Input: part model. Units: mm. Frame: model coordinates. A direction names the side the tool comes from. Round coordinates to 2 decimals unless told otherwise and drop trailing zeros. Loops run counter-clockwise (first coordinate to the right, second up) from the corner with the lowest first, then second, coordinate; pieces in that order, holes last. Notation, with made-up numbers: (29, -13.75) -> (83, -13.75) arc R13 ccw to (83, -9.75) -> close; hole circle Ø5 at (27.5, 13). An arc over 180 degrees is marked (long way). Answer as a JSON object with one key per item and string values. Group by question number.
Item 1: Set-up query: faces 1 (the flat face through (-53.68, -18.54, 1.06)), 2 (the flat face through (58, -6, 4.318)), 3 (the flat face through (-42, -6, 4.318)), 4 (the flat face through (58, -6, 0)). Return all of +Z, -Z, +X, -X, +Y, -Y with unobstructed straight access to the full face (end or side cutting, diameter ignored); none if empty.
Item 2: Material intervals for line 1 (Y direction, x = 51, z = 3); line 2 (Z direction, x = -2, y = -6.5); line 3 (X direction, y = -9, z = -0.5), sorted ascending. Write a range as [from, to].
Item 3: Pin query (flat end, axial travel): pin 1 (2 mm diameter, centred on y = -4.5, z = 4.5, fed in from -X); pin 2 (3.5 mm diameter, centred on x = 30.5, z = 2, fed in from -Y); pin 3 (4 mm diameter, centred on x = 8, y = -6.5, fed in from -Z). Return the tip coordinate at first contact, or that it passes through.
Item 4: Section query D-D on x = 54. Return loops of the section in (y, z), and give its area (3 significant figures).
Item 5: Draft query along X for faces 5 (the flat face through (30, -6, 6.096)), 6 (the flat face through (80.004, -11.053, 2.129)), 7 (the flat face through (4.6, -14.04, 1.06)). Return one class per face: released by +X, released by -X, zero draft, split by the parting line, or undercut.
from build123d import *

# Parameters (mm, degrees)
F2_DEPTH = 4.318
F3_SIZE  = 2.15899
F5_DEPTH = 1.778
F7_DEPTH = 1.778
F8_R     = 1.778
F9_SIZE  = 1.778


# Not quite as in the source:
# - a fillet or chamfer is up to 0.001 mm smaller than in the source, because OpenCascade refuses the exact size


with BuildPart() as f2:
    # F0 (on Top) → F2 (new body)
    with BuildSketch(Plane.XY):
        Polygon((27.5745280087, 3.6292271689), (27.5745280087, 1.2858584523), (27.5745280087, -13.2207097486), (27.5745280087, -15.5640784651), (32.4286483228, -15.5640784651), (32.4286483228, -13.3150536567), (32.4286483228, 1.3802023605), (32.4286483228, 3.6292271689), align=None)
        Polygon((72.2789242864, 1.3802023605), (32.4286483228, 1.3802023605), (32.4286483228, -13.3150536567), (72.2789242864, -13.3150536567), (75.0406160951, -15.9978345037), (85.1087123156, -5.9674256481), (75.0406160951, 4.0629832074), align=None)
        Polygon((-64.9878308177, 19.7724616155), (-86.7510214448, 19.7724616155), (-86.7510214448, -31.7073129117), (-64.9878308177, -31.7073129117), (-64.9878308177, -20.5603092909), (-42.1630144119, -18.7024753541), (-42.1630144119, -31.7073129117), (-15.7552305609, -31.7073129117), (-15.7552305609, -16.8446414173), (27.5745280087, -13.2207097486), (27.5745280087, 1.2858584523), (-15.7552305609, 4.909790121), (-15.7552305609, 19.7724616155), (-42.1630144119, 19.7724616155), (-42.1630144119, 6.7676240578), (-64.9878308177, 8.6254579946), align=None)
    extrude(amount=F2_DEPTH)

    # F3 (size 2.159 in the source; OpenCascade refuses exactly that, so slightly less here)
    f3_edges = [f2.edges().sort_by_distance(p)[0] for p in [
        (-53.575423, -19.631392, 4.318),
        (-42.163014, -25.204894, 4.318),
        (-28.959122, -31.707313, 4.318),
        (-15.755231, -24.275977, 4.318),
        (5.909649, -15.032676, 4.318),
        (5.909649, 3.097824, 4.318),
        (-15.755231, 12.341126, 4.318),
        (-28.959122, 19.772462, 4.318),
        (-42.163014, 13.270043, 4.318),
        (-53.575423, 7.696541, 4.318),
        (-64.987831, 14.19896, 4.318),
        (-75.869426, 19.772462, 4.318),
        (-86.751021, -5.967426, 4.318),
        (-75.869426, -31.707313, 4.318),
        (-64.987831, -26.133811, 4.318),
        (-28.959122, -31.707313, 0),
        (-15.755231, -24.275977, 0),
        (5.909649, -15.032676, 0),
        (-42.163014, -25.204894, 0),
        (-53.575423, -19.631392, 0),
        (-75.869426, -31.707313, 0),
        (-64.987831, -26.133811, 0),
        (-86.751021, -5.967426, 0),
        (-75.869426, 19.772462, 0),
        (-64.987831, 14.19896, 0),
        (-53.575423, 7.696541, 0),
        (-15.755231, 12.341126, 0),
        (5.909649, 3.097824, 0),
        (-42.163014, 13.270043, 0),
        (-28.959122, 19.772462, 0),
    ]]
    chamfer(f3_edges, length=F3_SIZE)

    # F4 (on face) → F5 (join)
    with BuildSketch(Plane.XY.offset(4.318)):
        Polygon((32.4286483228, 3.6292271689), (27.5745280087, 3.6292271689), (27.5745280087, 1.2858584523), (27.5745280087, -0.8806694518), (27.5745280087, -11.0541818444), (27.5745280087, -13.2207097486), (27.5745280087, -15.5640784651), (32.4286483228, -15.5640784651), (32.4286483228, -13.3150536567), (32.4286483228, 1.3802023605), align=None)
    extrude(amount=F5_DEPTH)

    # F6 (on face) → F7 (join)
    with BuildSketch(Plane(origin=(0, 0, 0), x_dir=(1, 0, 0), z_dir=(0, 0, -1))):
        Polygon((32.4286483228, 15.5640784651), (27.5745280087, 15.5640784651), (27.5745280087, 11.0541818444), (27.5745280087, 0.8806694518), (27.5745280087, -3.6292271689), (32.4286483228, -3.6292271689), (32.4286483228, -1.3802023605), (32.4286483228, 13.3150536567), align=None)
    extrude(amount=F7_DEPTH)

    # F8
    f8_edges = [f2.edges().sort_by_distance(p)[0] for p in [
        (52.353786, 1.380202, 0),
        (52.353786, -13.315054, 0),
        (52.353786, 1.380202, 4.318),
        (52.353786, -13.315054, 4.318),
    ]]
    fillet(f8_edges, radius=F8_R)

    # F9
    f9_edges = [f2.edges().sort_by_distance(p)[0] for p in [
        (30.001588, -15.564078, -1.778),
        (30.001588, -15.564078, 6.096),
        (30.001588, 3.629227, 6.096),
        (30.001588, 3.629227, -1.778),
    ]]
    chamfer(f9_edges, length=F9_SIZE)


solid = f2.part
Solved:
{
 "1": {"face 1": "-Z, -Y", "face 2": "+Z, +X, +Y, -Y", "face 3": "+Z, -X, +Y, -Y", "face 4": "-Z, +X, +Y, -Y"},
 "2": {"line 1": "[-13.25, 1.32]", "line 2": "[0, 4.32]", "line 3": "[27.57, 32.43]"},
 "3": {"pin 1": "x = -85.41", "pin 2": "y = -15.56", "pin 3": "z = 0"},
 "4": {"outline": "(-13.32, 1.78) arc R1.78 ccw to (-11.54, 0) -> (-0.4, 0) arc R1.78 ccw to (1.38, 1.78) -> (1.38, 2.54) arc R1.78 ccw to (-0.4, 4.32) -> (-11.54, 4.32) arc R1.78 ccw to (-13.32, 2.54) -> close", "area": "60.7 mm²"},
 "5": {"face 5": "zero draft", "face 6": "released by +X", "face 7": "undercut"}
}
